Can you work these out from the model? Positions are in its coordinate system, mm. A direction names the side the tool comes from. Round coordinates to 2 decimals unless told otherwise and drop trailing zeros. Loops run counter-clockwise (first coordinate to the right, second up) from the corner with the lowest first, then second, coordinate; pieces in that order, holes last. Notation, with made-up numbers: (74, -4.5) -> (89, -4.5) arc R20 cw to (89, 11.5) -> close; hole circle Ø2 at (71, -13). An arc over 180 degrees is marked (long way). Write each question's results on one line, items separated by ' | '.
from build123d import *

# Parameters (mm, degrees)
SKETCH1_W           = 40
SKETCH1_H           = 20
BOSS_EXTRUDE1_DEPTH = 20
SKETCH3_W           = 40
SKETCH3_H           = 20
BOSS_EXTRUDE2_DEPTH = 40
SKETCH4_W           = 30
SKETCH4_H           = 11.2
BOSS_EXTRUDE3_DEPTH = 10
SKETCH5_R           = 2
CUT_EXTRUDE1_DEPTH  = 35
SKETCH6_R           = 2
CUT_EXTRUDE2_DEPTH  = 35
FILLET2_R           = 2


with BuildPart() as part:
    # Sketch1 → Boss-Extrude1 (new body)
    with BuildSketch(Plane(origin=(0, 0, 0), x_dir=(1, 0, 0), z_dir=(0, 1, 0))):
        Rectangle(SKETCH1_W, SKETCH1_H)
    extrude(amount=-BOSS_EXTRUDE1_DEPTH)

    # Sketch3 → Boss-Extrude2 (add)
    with BuildSketch(Plane(origin=(0, 0, 0), x_dir=(1, 0, 0), z_dir=(0, 1, 0))):
        Rectangle(SKETCH3_W, SKETCH3_H)
    extrude(amount=BOSS_EXTRUDE2_DEPTH)

    # Sketch4 → Boss-Extrude3 (add)
    with BuildSketch(Plane.XZ.offset(20)):
        Rectangle(SKETCH4_W, SKETCH4_H)
    extrude(amount=BOSS_EXTRUDE3_DEPTH)

    # Sketch5 → Cut-Extrude1 (cut, symmetric)
    with BuildSketch(Plane(origin=(0, 0, -5.6), x_dir=(-1, 0, 0), z_dir=(0, 0, -1))):
        with Locations((0, -25)):
            Circle(SKETCH5_R)
        with Locations((12.5, -25)):
            Circle(SKETCH5_R)
        with Locations((-12.5, -25)):
            Circle(SKETCH5_R)
    extrude(amount=CUT_EXTRUDE1_DEPTH, both=True, mode=Mode.SUBTRACT)

    # Sketch6 → Cut-Extrude2 (cut)
    with BuildSketch(Plane(origin=(0, 0, -10), x_dir=(-1, 0, 0), z_dir=(0, 0, -1))):
        with Locations((12.5, 7.800844988)):
            Circle(SKETCH6_R)
        with Locations((12.5, 32.800844988)):
            Circle(SKETCH6_R)
        with Locations(Location((-12.5, 32.800844988, 0), (0, 0, 180))):
            Circle(SKETCH6_R)
        with Locations(Location((-12.5, 7.800844988, 0), (0, 0, 180))):
            Circle(SKETCH6_R)
    extrude(amount=-CUT_EXTRUDE2_DEPTH, mode=Mode.SUBTRACT)

    # Fillet2
    fillet2_edges = [part.edges().sort_by_distance(p)[0] for p in [
        (-20, 10, -10),
        (20, 10, -10),
        (20, 10, 10),
        (-20, 10, 10),
    ]]
    fillet(fillet2_edges, radius=FILLET2_R)


solid = part.part
1. If we section it at C-C (x = 0): List the corners of the cut face in (y, z) for me.
Final values:
outline: (-30, -5.6) -> (-27, -5.6) -> (-27, 5.6) -> (-30, 5.6) -> close; (-23, -5.6) -> (-20, -5.6) -> (-20, -10) -> (40, -10) -> (40, 10) -> (-20, 10) -> (-20, 5.6) -> (-23, 5.6) -> close
2. We'd pull the mould along Y, two halves only. Please class faces 1 (the face through (0, -20, -7)), 2 (the face through (10.9, 34, -0.1)), 3 (the face through (19.4, 10.42, 9.43)), 4 (the face through (0, 40, 0)): pulls with the +Y half, pulls with the -Y half, needs draft (parallel to the pull), parting line crosses it, or undercut.
Final values:
face 1: pulls with the -Y half | face 2: undercut | face 3: needs draft | face 4: pulls with the +Y half
3. If we section it at A-A (x = -12.5): List the corners of the cut face in (y, z) for me.
Final values:
outline: (-30, -5.6) -> (-27, -5.6) -> (-27, 5.6) -> (-30, 5.6) -> close; (-23, -5.6) -> (-20, -5.6) -> (-20, -10) -> (5.8, -10) -> (5.8, 10) -> (-20, 10) -> (-20, 5.6) -> (-23, 5.6) -> close; (9.8, -10) -> (30.8, -10) -> (30.8, 10) -> (9.8, 10) -> close; (34.8, -10) -> (40, -10) -> (40, 10) -> (34.8, 10) -> close
4. On a 3-axis mill with a long thin cutter (end or side, diameter ignored), from which of +Z, -Z, +X, -X, +Y, -Y can I reach the whole of each face in a straight line? I mean faces 5 (the face through (-15, -25, 0)), 6 (the face through (-11.026, 9.153, -0.14)), 7 (the face through (15, -25, 0)). Say none if no direction works.
Final values:
face 5: +Z, -Z, -X, -Y | face 6: +Z, -Z | face 7: +Z, -Z, +X, -Y
5. If we section it at D-D (x = -7.5): List the corners of the cut face in (y, z) for me.
Final values:
outline: (-30, -5.6) -> (-20, -5.6) -> (-20, -10) -> (40, -10) -> (40, 10) -> (-20, 10) -> (-20, 5.6) -> (-30, 5.6) -> close
6. Please list where these lines run through material, in increasing order: line 1 (Y direction, x = 12.5, z = -3.75); line 2 (Y direction, x = 14, z = 6.5); line 3 (Z direction, x = -2, y = -25.5). Write a range as from..to.
Final values:
line 1: -30..-27, -23..5.8, 9.8..30.8, 34.8..40 | line 2: -20..6.48, 9.12..31.48, 34.12..40 | line 3: -5.6..5.6
7. If we section it at B-B (y = -25): List the corners of the cut face in (x, z) for me, then the cut area to 3 significant figures.
Final values:
outline: (-15, -5.6) -> (-14.5, -5.6) -> (-14.5, 5.6) -> (-15, 5.6) -> close; (-10.5, -5.6) -> (-2, -5.6) -> (-2, 5.6) -> (-10.5, 5.6) -> close; (2, -5.6) -> (10.5, -5.6) -> (10.5, 5.6) -> (2, 5.6) -> close; (14.5, -5.6) -> (15, -5.6) -> (15, 5.6) -> (14.5, 5.6) -> close | area: 202 mm2
8. Will these pins go through, and if not, where does the flat tip stop? pin 1 (6.5 mm diameter, centred on x = 12.5, y = -25, fed in from +Z); pin 2 (11 mm diameter, centred on y = -27, z = 0, fed in from -X); pin 3 (5 mm diameter, centred on y = -26.5, z = 1, fed in from +X).
Final values:
pin 1: z = 5.6 | pin 2: x = -15 | pin 3: x = 15
